Here's how the part is built. I have some questions about the finished solid (model axes, mm). Face numbers are marked on the shaded views. A direction names the side the tool comes from. Coordinates: 2 decimals unless noted, no trailing zeros. Loops run counter-clockwise (first coordinate to the right, second up) from the corner with the lowest first, then second, coordinate; pieces in that order, holes last. Notation, with made-up numbers: (49, -23.5) -> (79, -23.5) arc R13 cw to (79, -1.5) -> close; hole circle Ø11 at (62, 49). An arc over 180 degrees is marked (long way). Answer as a JSON object with one key per item and string values. Group by question number.
Q1. I want a section at D-D on z = 3.5. Write out the boundary of the cut face in (x, y).
Q2. I'm going to push flat-ended pins straight in: pin 1 (3 mm diameter, centred on x = 9, z = 4, fed in from +Y); pin 2 (4 mm diameter, centred on x = -3.5, z = 3.5, fed in from +Y); pin 3 (4 mm diameter, centred on y = -2, z = 3, fed in from -X). Where does each tip first touch, or does it pass through?
Q3. Thinking about a two-plate mould opening in X: for the marked faces 4 and 5, which applies, released by +X, released by -X, zero draft, split by the parting line, or undercut?
Q4. I want a section at C-C on z = 5.5. Write out the boundary of the cut face in (x, y), then the cut area to 3 significant figures.
Q5. On a 3-axis mill with a long thin cutter (end or side, diameter ignored), from which of +Z, -Z, +X, -X, +Y, -Y can I reach the whole of each face in a straight line? I mean the marked faces 1, 2 and 3. Say none if no direction works.
Q6. I need wall thicknesses on line 1 (Z direction, x = 3.5, y = 11); line 2 (Y direction, x = 0, z = 4.75); line 3 (Y direction, x = 2.5, z = 6.25). Which ranges of each line are inside material? Lowest first, please.
```python
from build123d import *

# Parameters (mm, degrees)
SKETCH_1_R          = 13.7
EXTRUDE_1_DEPTH     = 8
SKETCH_4_R          = 5
CUT_EXTRUDE_1_DEPTH = 21.961393083
EXTRUDE_2_REACH     = 25.034
SKETCH_5_W          = 7.968626967
SKETCH_5_H          = 13.552288672


with BuildPart() as part:
    # 스케치1 → 보스-돌출1 (new body)
    with BuildSketch(Plane.XY):
        Circle(SKETCH_1_R)
    extrude(amount=EXTRUDE_1_DEPTH)

    # 스케치2 → 컷-회전1 (revolve, cut)
    with BuildSketch(Plane(origin=(0, 0, 0), x_dir=(1, 0, 0), z_dir=(0, 1, 0)), mode=Mode.PRIVATE) as cut_revolve_1_sk:
        with BuildLine():
            Line((-14.7, 0), (-14.7, -8))
            Line((-14.7, -8), (-14.2, -8))
            ThreePointArc((-14.2, -8), (-10.2, -4), (-14.2, 0))
            Line((-14.2, 0), (-14.7, 0))
        make_face()
    revolve(cut_revolve_1_sk.sketch.rotate(Axis((0, 0, 12.586575048), (0, 0, -1)), 180), axis=Axis((0, 0, 12.586575048), (0, 0, -1)), mode=Mode.SUBTRACT)

    # 스케치4 → 컷-돌출1 (cut, through all)
    with BuildSketch(Plane(origin=(0, 0, 0), x_dir=(-1, 0, 0), z_dir=(0, 0, -1))):
        Circle(SKETCH_4_R)
    extrude(amount=-CUT_EXTRUDE_1_DEPTH, mode=Mode.SUBTRACT)

    # 스케치5 → 보스-돌출2 (add, up to next)
    with BuildSketch(Plane(origin=(3, 0, 0), x_dir=(0, 0, -1), z_dir=(1, 0, 0)), mode=Mode.PRIVATE) as extrude_2_sk1:
        with Locations((-3.984313484, -0.077510512)):
            Rectangle(SKETCH_5_W, SKETCH_5_H)
    extrude_2_tool1 = extrude(extrude_2_sk1.sketch, amount=EXTRUDE_2_REACH, mode=Mode.PRIVATE) - part.part
    add(extrude_2_tool1.solids().sort_by_distance((3, -0.077511, 3.984313))[0])


solid = part.part
```
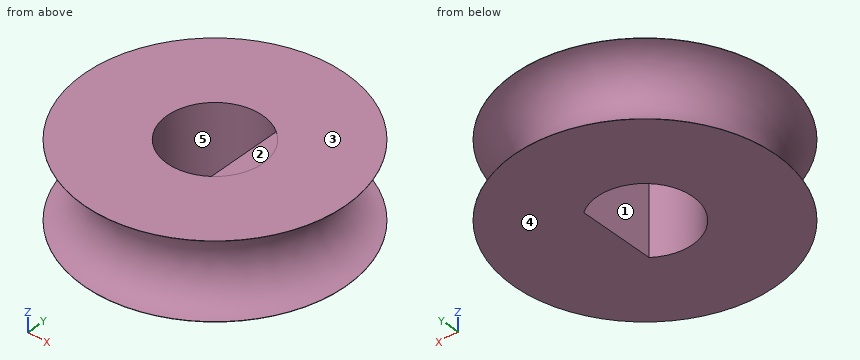
Result set:
{
 "1": {"outline": "circle Ø20.46 at (0, 0); hole (3, -4) -> (3, 4) arc R5 ccw (long way) to start"},
 "2": {"pin 1": "stops at y = 6.91", "pin 2": "stops at y = 10.62", "pin 3": "stops at x = -11.4"},
 "3": {"face 4": "zero draft", "face 5": "undercut"},
 "4": {"outline": "circle Ø20.98 at (0, 0); hole (3, -4) -> (3, 4) arc R5 ccw (long way) to start", "area": "278 mm²"},
 "5": {"face 1": "+Z, -Z", "face 2": "+Z", "face 3": "+Z, +X, -X, +Y, -Y"},
 "6": {"line 1": "z = 0 to 1.01, 6.99 to 8", "line 2": "y = -10.27 to -5, 5 to 10.27", "line 3": "y = -10.6 to -4.33, 4.33 to 10.6"}
}
